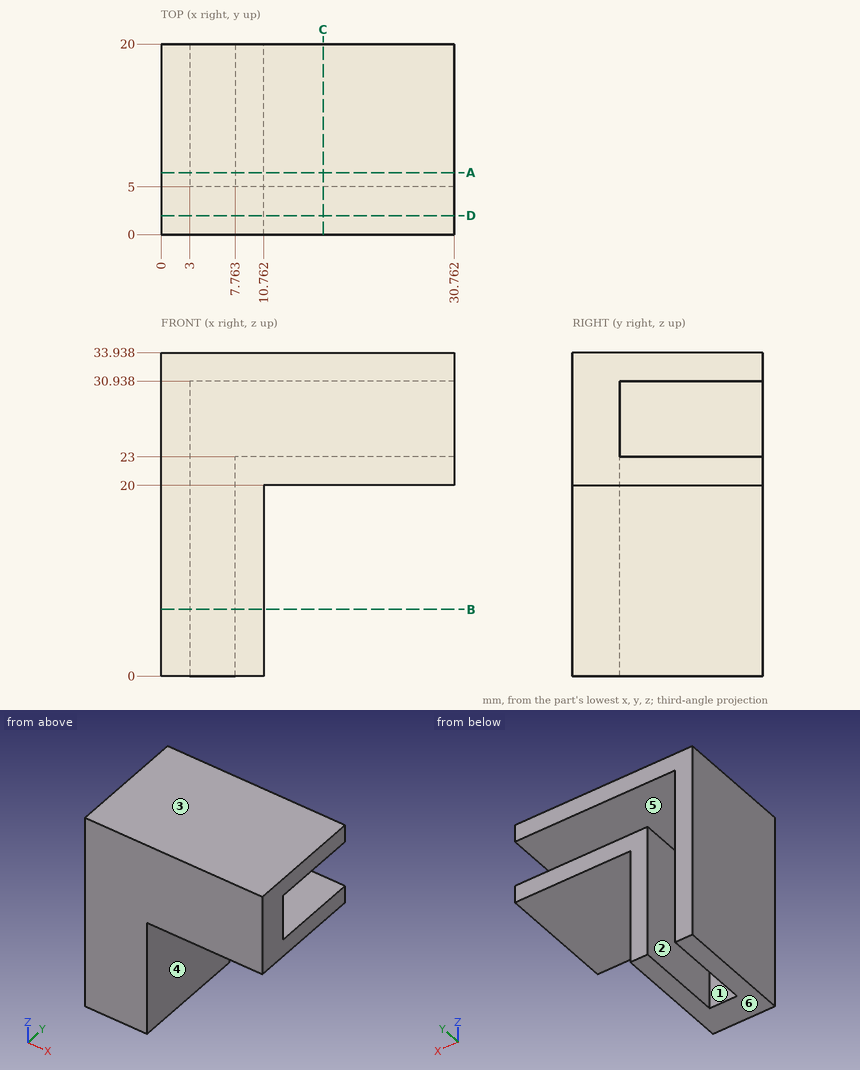
Geometry: see drawing. Coordinates: mm, zero at the bounding-box minimum. A direction names the side the tool comes from. Round coordinates to 2 decimals unless told otherwise and drop trailing zeros. Write each loop counter-clockwise with the first axis right and the second up, starting at its lowest first coordinate (ties: lowest second). Pieces come first, ordered by that corner, then holes. Notation, with made-up numbers: M 58.5,6 L 87.5,6 A23 ccw 87.5,14 Z; hole C -9,-3 d11. An arc over 180 degrees is marked long. Answer in a Markdown table with one row per item. Add a question column.
(1) Cut plane D-D, the plane y = 2. Return the cut outline in (x, z).
(2) Reachability of the marked faces 4, 5 and 6 from +Z, -Z, +X, -X, +Y, -Y: full face, straight path, thin tool, end or side. Return the list, or none.
(3) Cut plane B-B, the plane z = 7. Return the cut outline in (x, y).
(4) Ray query, L1, parallel to X at y = 17, z = 20.5; L2, parallel to X at y = 16.5, z = 11.5; L3, parallel to Z at x = 14, y = 9. Return the intervals inside material, ascending.
(5) Cut plane C-C, the plane x = 17. Return the cut outline in (y, z).
(6) Draft query along Z for the marked faces 1, 2 and 3. Return one class per face: pulls with the +Z half, pulls with the -Z half, needs draft (parallel to the pull), parting line crosses it, or undercut.
(7) Contact query for flat-ended pins moving along their axis: pin 1 (2 mm diameter, centred on x = 25, y = 15.5, fed in from -Z); pin 2 (2 mm diameter, centred on y = 12.5, z = 25, fed in from +X); pin 3 (6 mm diameter, centred on x = 11.5, z = 23, fed in from -Y); pin 4 (3 mm diameter, centred on y = 16, z = 6.5, fed in from +X). Output: stop coordinate, or through.
(8) Cut plane A-A, the plane y = 6.5. Return the cut outline in (x, z), then the cut area to 3 significant figures.
Established:
| question | item | result |
|---|---|---|
| 1 | outline | M 0,0 L 10.76,0 L 10.76,20 L 30.76,20 L 30.76,33.94 L 0,33.94 Z |
| 2 | face 4 | -Z, +X, +Y, -Y |
| 2 | face 5 | +X, +Y |
| 2 | face 6 | -Z, +X, -X, +Y, -Y |
| 3 | outline | M 0,0 L 10.76,0 L 10.76,20 L 7.76,20 L 7.76,5 L 3,5 L 3,20 L 0,20 Z |
| 4 | L1 | 0 to 3, 7.76 to 30.76 |
| 4 | L2 | 0 to 3, 7.76 to 10.76 |
| 4 | L3 | 20 to 23, 30.94 to 33.94 |
| 5 | outline | M 0,20 L 20,20 L 20,23 L 5,23 L 5,30.94 L 20,30.94 L 20,33.94 L 0,33.94 Z |
| 6 | face 1 | undercut |
| 6 | face 2 | needs draft |
| 6 | face 3 | pulls with the +Z half |
| 7 | pin 1 | z = 20 |
| 7 | pin 2 | x = 3 |
| 7 | pin 3 | y = 0 |
| 7 | pin 4 | x = 10.76 |
| 8 | outline | M 0,0 L 3,0 L 3,30.94 L 30.76,30.94 L 30.76,33.94 L 0,33.94 Z; M 7.76,0 L 10.76,0 L 10.76,20 L 30.76,20 L 30.76,23 L 7.76,23 Z |
| 8 | area | 314 mm² |
